Input: part model. Units: mm. Frame: model coordinates. A direction names the side the tool comes from. Coordinates: 2 decimals unless noted, no trailing zeros. Write each loop counter-clockwise with the first axis right and the second up, starting at its lowest first coordinate (ties: lowest second). Pieces come first, ordered by that corner, then holes.
1) Section query A-A (z = 6.25). State how many separate pieces and enclosed holes the cut face has, then the cut area to 3 significant figures.
2) Set-up query: faces 5 (the flat face through (-11.45, 0, 8)), 6 (the cylindrical face through (9.38, -4.6, 9.1)). Return all of +Z, -Z, +X, -X, +Y, -Y with unobstructed straight access to the full face (end or side cutting, diameter ignored); none if empty.
3) Section query D-D (x = 0.5). Output: boundary loops of the cut face in (y, z), then the cut area to 3 significant figures.
4) Section query C-C (y = -4.25). Output: boundary loops of the cut face in (x, z).
5) Draft query along Y for faces 1 (the flat face through (0, -6.7, 8)), 2 (the flat face through (-4, 3.2, 4)), 3 (the cylindrical face through (9.35, 4.63, 9.1)), 4 (the flat face through (0, 6.7, 8)). Return one class per face: pulls with the +Y half, pulls with the -Y half, needs draft (parallel to the pull), parting line crosses it, or undercut.
6) Section query B-B (x = -5.25). Output: boundary loops of the cut face in (y, z).
7) Line query: L1, parallel to X at y = -0.5, z = 10.5; L2, parallel to Y at x = 4.5, z = 3.75; L3, parallel to Y at x = 3.75, z = 6.25. Output: solid intervals per line, ascending.
8) Pin query (flat end, axial travel): pin 1 Ø2.5 at (x, y) = (5, 1.5) entering from +Z; pin 2 Ø0.7 at (x, y) = (-4, 2.5) entering from +Z. Return the tip coordinate at first contact, or that it passes through.
from build123d import *

# Parameters (mm, degrees)
F0_W     = 22.9
F0_H     = 13.4
F1_DEPTH = 2
F2_W     = 22.9
F2_H     = 13.4
F2_W_2   = 19.9
F2_H_2   = 10.4
F3_DEPTH = 14
F4_W     = 15.9
F4_H     = 6.4
F5_DEPTH = 12
F6_W     = 7.6
F6_H     = 1.698620432
F6_W_2   = 4.9
F7_DEPTH = 8
F8_W     = 3.4
F8_H     = 6.4
F9_DEPTH = 4
F10_SIZE = 0.5
F11_R    = 2


with BuildPart() as f1:
    # F0 (on Top) → F1 (new body)
    with BuildSketch(Plane.XY):
        Rectangle(F0_W, F0_H)
    extrude(amount=F1_DEPTH)

    # F2 (on face) → F3 (join)
    with BuildSketch(Plane.XY.offset(2)):
        Rectangle(F2_W, F2_H)
        Rectangle(F2_W_2, F2_H_2, mode=Mode.SUBTRACT)
    extrude(amount=F3_DEPTH)

    # F4 (on face) → F5 (join)
    with BuildSketch(Plane.XY.offset(2)):
        Rectangle(F4_W, F4_H)
    extrude(amount=F5_DEPTH)

    # F6 (on face) → F7 (cut)
    with BuildSketch(Plane.XY.offset(14)):
        with Locations((-4.15, 2.350689784)):
            Rectangle(F6_W, F6_H)
        Polygon((-0.35, 3.2), (-0.35, 1.501379568), (-0.35, -3.2), (3.05, -3.2), (3.05, 1.501379568), (3.05, 3.2), align=None)
        with Locations((5.5, 2.350689784)):
            Rectangle(F6_W_2, F6_H)
    extrude(amount=-F7_DEPTH, mode=Mode.SUBTRACT)

    # F8 (on face) → F9 (cut)
    with BuildSketch(Plane.XY.offset(6)):
        with Locations((1.35, 0)):
            Rectangle(F8_W, F8_H)
    extrude(amount=-F9_DEPTH, mode=Mode.SUBTRACT)

    # F10
    f10_edges = [f1.edges().sort_by_distance(p)[0] for p in [
        (-4.15, 1.50138, 14),
        (-0.35, -0.84931, 14),
        (-4.15, -3.2, 14),
        (-7.95, -0.84931, 14),
        (-7.95, 1.50138, 10),
        (-0.35, 1.50138, 10),
        (-0.35, -3.2, 8),
        (3.05, -3.2, 8),
        (7.95, -0.84931, 14),
        (5.5, -3.2, 14),
        (3.05, -0.84931, 14),
        (5.5, 1.50138, 14),
        (7.95, 1.50138, 10),
        (3.05, 1.50138, 10),
        (3.05, 3.2, 4),
        (7.95, 3.2, 4),
        (7.95, -3.2, 8),
        (-0.35, 3.2, 4),
        (-7.95, 3.2, 4),
        (-7.95, -3.2, 8),
    ]]
    chamfer(f10_edges, length=F10_SIZE)

    # F11
    f11_edges = [f1.edges().sort_by_distance(p)[0] for p in [
        (9.95, -5.2, 9),
        (9.95, 5.2, 9),
        (-9.95, 5.2, 9),
        (-9.95, -5.2, 9),
        (11.45, -6.7, 8),
        (11.45, 6.7, 8),
        (-11.45, 6.7, 8),
        (-11.45, -6.7, 8),
    ]]
    fillet(f11_edges, radius=F11_R)


solid = f1.part
Answer:
1. separate pieces: 3
1. enclosed holes: 1
1. area: 158 mm2
2. face 5: +Z, -Z, -X, +Y, -Y
2. face 6: +Z
3. outline: (-6.7, 0) - (6.7, 0) - (6.7, 16) - (5.2, 16) - (5.2, 2) - (-5.2, 2) - (-5.2, 16) - (-6.7, 16) - close
3. area: 68.8 mm2
4. outline: (-11.45, 0) - (11.45, 0) - (11.45, 16) - (9.65, 16) - (9.65, 2) - (-9.65, 2) - (-9.65, 16) - (-11.45, 16) - close
5. face 1: pulls with the -Y half
5. face 2: undercut
5. face 3: undercut
5. face 4: pulls with the +Y half
6. outline: (-6.7, 0) - (6.7, 0) - (6.7, 16) - (5.2, 16) - (5.2, 2) - (3.2, 2) - (3.2, 6) - (1.5, 6) - (1.5, 13.5) - (1, 14) - (-2.7, 14) - (-3.2, 13.5) - (-3.2, 2) - (-5.2, 2) - (-5.2, 16) - (-6.7, 16) - close
7. L1: x = -11.45 to -9.95, -7.95 to -0.35, 3.05 to 7.95, 9.95 to 11.45
7. L2: y = -6.7 to -5.2, -3.2 to 3.2, 5.2 to 6.7
7. L3: y = -6.7 to -5.2, -3.2 to 1.5, 5.2 to 6.7
8. pin 1: stops at z = 14
8. pin 2: stops at z = 6
